```python
from build123d import *

# Parameters (mm, degrees)
SKETCH_1_W          = 49
SKETCH_1_H          = 26
SKETCH_1_R          = 5.1
EXTRUDE_1_DEPTH     = 3
SKETCH_5_W          = 3
SKETCH_5_H          = 12
EXTRUDE_2_DEPTH     = 3
SKETCH_2_W          = 12
SKETCH_2_H          = 3
EXTRUDE_3_DEPTH     = 3
SKETCH_8_R          = 1
CUT_EXTRUDE_5_DEPTH = 32.957002363
FILLET_1_R          = 10
SKETCH_6_W          = 12.982120022
SKETCH_6_H          = 9.5
SKETCH_6_H_2        = 6.5
CUT_EXTRUDE_3_DEPTH = 32.957002363
FILLET_2_R          = 2


with BuildPart() as part:
    # 草图1 → 凸台-拉伸1 (new body)
    with BuildSketch(Plane(origin=(0, 0, 0), x_dir=(1, 0, 0), z_dir=(0, 1, 0))):
        Rectangle(SKETCH_1_W, SKETCH_1_H)
        with Locations(Location((0.5, 2, 0), (0, 0, 270))):
            Circle(SKETCH_1_R, mode=Mode.SUBTRACT)
    extrude(amount=EXTRUDE_1_DEPTH)

    # 草图5 → 凸台-拉伸2 (add)
    with BuildSketch(Plane.XZ):
        with Locations((-26, 2)):
            Rectangle(SKETCH_5_W, SKETCH_5_H)
    extrude(amount=-EXTRUDE_2_DEPTH)

    # 草图2 → 凸台-拉伸3 (add)
    with BuildSketch(Plane(origin=(0, 3, 0), x_dir=(1, 0, 0), z_dir=(0, 1, 0))):
        with Locations((-14, -14.5)):
            Rectangle(SKETCH_2_W, SKETCH_2_H)
        with Locations((14, -14.5)):
            Rectangle(SKETCH_2_W, SKETCH_2_H)
    extrude(amount=-EXTRUDE_3_DEPTH)

    # 草图8 → 切除-拉伸5 (cut, through all)
    with BuildSketch(Plane(origin=(0, 3, 0), x_dir=(1, 0, 0), z_dir=(0, 1, 0))):
        with Locations((21, -13)):
            Circle(SKETCH_8_R)
        with Locations((7, -13)):
            Circle(SKETCH_8_R)
        with Locations((-7, -13)):
            Circle(SKETCH_8_R)
        with Locations((-21, -13)):
            Circle(SKETCH_8_R)
        with Locations((-24.5, -9)):
            Circle(SKETCH_8_R)
        with Locations((-24.5, 5)):
            Circle(SKETCH_8_R)
    extrude(amount=-CUT_EXTRUDE_5_DEPTH, mode=Mode.SUBTRACT)

    # 圆角1
    fillet_1_edges = [part.edges().sort_by_distance(p)[0] for p in [
        (24.5, 1.5, -13),
    ]]
    fillet(fillet_1_edges, radius=FILLET_1_R)

    # 草图6 → 切除-拉伸3 (cut, through all)
    with BuildSketch(Plane(origin=(0, 3, 0), x_dir=(1, 0, 0), z_dir=(0, 1, 0))):
        with Locations((-13.991060011, -4.25)):
            Rectangle(SKETCH_6_W, SKETCH_6_H)
        with Locations((-13.991060011, 6.75)):
            Rectangle(SKETCH_6_W, SKETCH_6_H_2)
        with Locations((14.991060011, -4.25)):
            Rectangle(SKETCH_6_W, SKETCH_6_H)
        with BuildLine():
            Line((8.5, 3.5), (8.5, 10))
            Line((8.5, 10), (14.5, 10))
            ThreePointArc((14.5, 10), (19.269696007, 8.123475383), (21.482120022, 3.5))
            Line((21.482120022, 3.5), (8.5, 3.5))
        make_face()
    extrude(amount=-CUT_EXTRUDE_3_DEPTH, mode=Mode.SUBTRACT)

    # 圆角2
    fillet_2_edges = [part.edges().sort_by_distance(p)[0] for p in [
        (-20.482120022, 1.5, -3.5),
        (-20.482120022, 1.5, -10),
        (-7.5, 1.5, -10),
        (-7.5, 1.5, -3.5),
        (21.482120022, 1.5, -0.5),
        (21.482120022, 1.5, 9),
        (8.5, 1.5, 9),
        (8.5, 1.5, -0.5),
        (8.5, 1.5, -10),
        (21.482120022, 1.5, -3.5),
        (8.5, 1.5, -3.5),
        (-20.482120022, 1.5, 9),
        (-20.482120022, 1.5, -0.5),
        (-7.5, 1.5, -0.5),
        (-7.5, 1.5, 9),
    ]]
    fillet(fillet_2_edges, radius=FILLET_2_R)


solid = part.part
```
CAD build for the part. Positions are in the model's coordinates, mm. A direction names the side the tool comes from. Round coordinates to 2 decimals unless told otherwise and drop trailing zeros. Order: outer loops, then holes, each group sorted by start corner. A loop starts at its lowest first (then second) coordinate and runs counter-clockwise, first axis right, second up. Notation, with made-up numbers: (-15, -9.75) - (14, -9.75) arc R25 cw to (14, 14.25) - close; hole circle Ø5 at (87.5, 84). An arc over 180 degrees is marked (long way). Use CSV: the item, a comma, the result in double quotes. Start each with the question number.
1) Saw through at C-C (x = 0.5). List the corners of the cut face in (y, z), and give its area (3 significant figures).
2) Pin check, flat tips, straight feed: pin 1 Ø1.2 at (y, z) = (1, -6) entering from +X; pin 2 Ø1.5 at (y, z) = (1.5, 11.5) entering from -X; pin 3 Ø6 at (x, z) = (0.5, -2) entering from +Y; pin 4 Ø1.5 at (y, z) = (1.5, 14) entering from +X. Stop position of each tip, or through.
3) Two-plate mould, pull along X, no slides. Class faces 5 (the flat face through (15, 2, -0.5)), 6 (the flat face through (-26, 1, -4)), 7 (the cylindrical face through (21.65, 1.52, -9.99)): pulls with the +X half, pulls with the -X half, needs draft (parallel to the pull), parting line crosses it, or undercut.
4) Saw through at A-A (x = -16). List the corners of the cut face in (y, z).
5) Saw through at D-D (z = 2). List the corners of the cut face in (x, y), and give its area (3 significant figures).
6) Tool access for faces 1 (the cylindrical face through (-19.88, 1.48, 8.43)), 2 (the flat face through (23, 1, 13)), 3 (the flat face through (-20, 2, 15)), 4 (the cylindrical face through (-23.5, 1.5, -5)): list every direction of +Z, -Z, +X, -X, +Y, -Y with a clear straight run to the whole face (end or side of a thin tool).
7) Saw through at B-B (z = -2). List the corners of the cut face in (x, y), and give its area (3 significant figures).
8) Wall check: L1, parallel to X at y = 2, z = 3.25; L2, parallel to Z at x = -11, y = 1.3; L3, parallel to X at y = 1.65, z = -2. Give the ranges that are in metal, low to high. Write a range as [from, to].
Values follow:
1,outline,"(0, -13) - (3, -13) - (3, -7.1) - (0, -7.1) - close; (0, 3.1) - (3, 3.1) - (3, 13) - (0, 13) - close"
1,area,"47.4 mm2"
2,pin 1,"stops at x = 24.21"
2,pin 2,"stops at x = -24.5"
2,pin 3,"passes through"
2,pin 4,"stops at x = 20"
3,face 5,"undercut"
3,face 6,"needs draft"
3,face 7,"pulls with the +X half"
4,outline,"(0, -13) - (3, -13) - (3, -10) - (0, -10) - close; (0, -3.5) - (3, -3.5) - (3, -0.5) - (0, -0.5) - close; (0, 9) - (3, 9) - (3, 16) - (0, 16) - close"
5,outline,"(-27.5, 0) - (-20.48, 0) - (-20.48, 3) - (-27.5, 3) - close; (-7.5, 0) - (-2.66, 0) - (-2.66, 3) - (-7.5, 3) - close; (3.66, 0) - (8.5, 0) - (8.5, 3) - (3.66, 3) - close; (21.48, 0) - (24.5, 0) - (24.5, 3) - (21.48, 3) - close"
5,area,"59.1 mm2"
6,face 1,"+Y, -Y"
6,face 2,"+Z, +X, +Y, -Y"
6,face 3,"+Z, -X, +Y, -Y"
6,face 4,"-X, +Y, -Y"
7,outline,"(-27.5, 0) - (-4.6, 0) - (-4.6, 3) - (-27.5, 3) - close; (5.6, 0) - (24.5, 0) - (24.5, 3) - (5.6, 3) - close"
7,area,"125 mm2"
8,L1,"x = [-27.5, -20.48], [-7.5, 8.5], [21.48, 24.5]"
8,L2,"z = [-13, -10], [-3.5, -0.5], [9, 16]"
8,L3,"x = [-27.5, -4.6], [5.6, 24.5]"
